from build123d import *

# Parameters (mm, degrees)
SKETCH1_R           = 4.5
SKETCH1_R_2         = 2
BOSS_EXTRUDE1_DEPTH = 11
BOSS_EXTRUDE2_START = 11
SKETCH1_3_W         = 9.6
SKETCH1_3_H         = 9.6
SKETCH1_3_R         = 4.5
SKETCH1_3_R_2       = 2
BOSS_EXTRUDE2_DEPTH = 6.4
BOSS_EXTRUDE3_START = 17.4
SKETCH1_4_R         = 7.3
SKETCH1_4_W         = 9.6
SKETCH1_4_H         = 9.6
SKETCH1_4_R_2       = 4.5
SKETCH1_4_R_3       = 2
BOSS_EXTRUDE3_DEPTH = 4
CUT_EXTRUDE1_START  = 21.4
SKETCH1_5_R         = 2
CUT_EXTRUDE1_DEPTH  = 10


with BuildPart() as part:
    # Sketch1 → Boss-Extrude1 (new body)
    with BuildSketch(Plane(origin=(0, 0, 0), x_dir=(1, 0, 0), z_dir=(0, 1, 0))):
        Circle(SKETCH1_R)
        Circle(SKETCH1_R_2, mode=Mode.SUBTRACT)
        Circle(SKETCH1_R_2)
    extrude(amount=BOSS_EXTRUDE1_DEPTH)

    # Sketch1<3> → Boss-Extrude2 (add)
    with BuildSketch(Plane(origin=(0, 0, 0), x_dir=(1, 0, 0), z_dir=(0, 1, 0)).offset(BOSS_EXTRUDE2_START)):
        Rectangle(SKETCH1_3_W, SKETCH1_3_H)
        Circle(SKETCH1_3_R, mode=Mode.SUBTRACT)
        Circle(SKETCH1_3_R)
        Circle(SKETCH1_3_R_2, mode=Mode.SUBTRACT)
        Circle(SKETCH1_3_R_2)
    extrude(amount=BOSS_EXTRUDE2_DEPTH)

    # Sketch1<4> → Boss-Extrude3 (add)
    with BuildSketch(Plane(origin=(0, 0, 0), x_dir=(1, 0, 0), z_dir=(0, 1, 0)).offset(BOSS_EXTRUDE3_START)):
        Circle(SKETCH1_4_R)
        Rectangle(SKETCH1_4_W, SKETCH1_4_H, mode=Mode.SUBTRACT)
        Rectangle(SKETCH1_4_W, SKETCH1_4_H)
        Circle(SKETCH1_4_R_2, mode=Mode.SUBTRACT)
        Circle(SKETCH1_4_R_2)
        Circle(SKETCH1_4_R_3, mode=Mode.SUBTRACT)
        Circle(SKETCH1_4_R_3)
    extrude(amount=BOSS_EXTRUDE3_DEPTH)

    # Sketch1<5> → Cut-Extrude1 (cut)
    with BuildSketch(Plane(origin=(0, 0, 0), x_dir=(1, 0, 0), z_dir=(0, 1, 0)).offset(CUT_EXTRUDE1_START)):
        Circle(SKETCH1_5_R)
    extrude(amount=-CUT_EXTRUDE1_DEPTH, mode=Mode.SUBTRACT)


solid = part.part
Work out the finished part from the listing and answer in its coordinate system (mm). A direction names the side the tool comes from. Round coordinates to 2 decimals unless told otherwise and drop trailing zeros. Loops run counter-clockwise (first coordinate to the right, second up) from the corner with the lowest first, then second, coordinate; pieces in that order, holes last. Notation, with made-up numbers: (46.25, 4.5) - (80.25, 4.5) arc R27 ccw to (80.25, 23.5) - close; hole circle Ø4 at (16.25, 87). An arc over 180 degrees is marked (long way). One line per item, written item: value.
Q1. Find section B-B on y = 14.75. Give the vertices of the cut face in (x, z).
Check values:
outline: (-4.8, -4.8) - (4.8, -4.8) - (4.8, 4.8) - (-4.8, 4.8) - close; hole circle Ø4 at (0, 0)
Q2. Straight lines are drawn through the part: probe 1 along X at (y, z) = (16, 0); probe 2 along Y at (x, z) = (5.75, 3.75). For each, find the intervals that lie inside material, in ascending order.
Check values:
probe 1: -4.8 to -2, 2 to 4.8
probe 2: 17.4 to 21.4
Q3. For faces 4 (the flat face through (0, 14, 4.8)), 5 (the flat face through (4.8, 14, 0)), 6 (the flat face through (0, 14, -4.8)), 7 (the flat face through (-4.8, 14, 0)), determine the directions among +Z, -Z, +X, -X, +Y, -Y from which every point of the face is accessible in a straight line to the end or side of a thin tool.
Check values:
face 4: +Z, +X, -X, -Y
face 5: +Z, -Z, +X, -Y
face 6: -Z, +X, -X, -Y
face 7: +Z, -Z, -X, -Y
Q4. Find section C-C on z = 0. Give the vertices of the cut face in (x, y), and give its area (3 significant figures).
Check values:
outline: (-7.3, 17.4) - (-4.8, 17.4) - (-4.8, 11) - (-4.5, 11) - (-4.5, 0) - (4.5, 0) - (4.5, 11) - (4.8, 11) - (4.8, 17.4) - (7.3, 17.4) - (7.3, 21.4) - (2, 21.4) - (2, 11.4) - (-2, 11.4) - (-2, 21.4) - (-7.3, 21.4) - close
area: 179 mm2
Q5. Find section A-A on x = 0. Give the vertices of the cut face in (y, z), and give its area (3 significant figures).
Check values:
outline: (0, -4.5) - (11, -4.5) - (11, -4.8) - (17.4, -4.8) - (17.4, -7.3) - (21.4, -7.3) - (21.4, -2) - (11.4, -2) - (11.4, 2) - (21.4, 2) - (21.4, 7.3) - (17.4, 7.3) - (17.4, 4.8) - (11, 4.8) - (11, 4.5) - (0, 4.5) - close
area: 179 mm2
Q6. Each of these flat-tipped pins is pushed along its axis until it touches: pin 1 Ø3 at (x, z) = (1.5, 0) entering from -Y; pin 2 Ø3 at (x, y) = (-0.5, 14) entering from +Z; pin 3 Ø3 at (y, z) = (6, 3.5) entering from -X; pin 4 Ø5 at (y, z) = (14, 1) entering from -X. Where does it stop, or does it pass through?
Check values:
pin 1: y = 0
pin 2: z = 4.8
pin 3: x = -4.03
pin 4: x = -4.8
Q7. The mould has two halves that part along Z. Classify faces 1 (the cylindrical face through (6.963, 19.372, -2.193)), 2 (the flat face through (0, 0, 0)), 3 (the cylindrical face through (0, 16, 2)): +Z half, -Z half, draft (parallel to the pull), parting line (faces both ways), or undercut.
Check values:
face 1: parting line
face 2: draft
face 3: undercut
Q8. Find section D-D on y = 10.25. Give the vertices of the cut face in (x, z), and give its area (3 significant figures).
Check values:
outline: circle Ø9 at (0, 0)
area: 63.6 mm2
